Read the model definition and answer for the solid it produces. Units are mm, in the model's axes. A direction names the side the tool comes from. Coordinates: 2 decimals unless noted, no trailing zeros. Write each loop counter-clockwise with the first axis right and the second up, starting at its lowest first coordinate (ties: lowest second). Pieces come first, ordered by that corner, then holes.
1) Determine the mould class of faces 1 (the face through (0, 11, -17.5)), 2 (the face through (15.32, 3.62, 13.75)), 3 (the face through (-4.29, 13, 15)), 4 (the face through (-15, 13, 10.015)) for opening direction X: +X half, -X half, draft (parallel to the pull), parting line (faces both ways), or undercut.
2) The part is cut by section D-D (y = 13). Determine the outline of the cut face in (x, z), then the cut area to 3 significant figures.
3) The part is cut by section C-C (x = 4). Determine the outline of the cut face in (y, z).
4) Each of these flat-tipped pins is pushed along its axis until it touches: pin 1 Ø2.5 at (x, z) = (-15.25, 15.25) entering from +Y (3 decimals); pin 2 Ø1.8 at (x, y) = (-19, 0.5) entering from -Z; pin 3 Ø1 at (y, z) = (13, -15.5) entering from +X; pin 4 Ø0.6 at (x, y) = (-6.5, 1) entering from +Z. Where does it stop, or does it pass through?
5) Find the intervals of material crossed by line 1 (X direction, y = 8.75, z = 15.25); line 2 (Y direction, x = 18, z = 14); line 3 (Y direction, x = 5, z = -9), in increasing order.
6) Which of the six approach directions +Z, -Z, +X, -X, +Y, -Y give full straight-line access (tool end or side, diameter ignored) to faces 5 (the face through (-19, 1, -15.25)), 6 (the face through (1, 13, -0.479)), 7 (the face through (1, 13, -10.493)), 8 (the face through (-13.972, 13, 7)), 9 (the face through (-9, 13, 13.604))?
7) The part is cut by section B-B (z = -3). Determine the outline of the cut face in (x, y), then the cut area to 3 significant figures.
8) The part is cut by section A-A (y = 4). Determine the outline of the cut face in (x, z), then the cut area to 3 significant figures.
from build123d import *

# Parameters (mm, degrees)
EXTRUDE_1_DEPTH     = 2
SKETCH_2_R          = 2.5
EXTRUDE_2_DEPTH     = 5
EXTRUDE_START       = 8
SKETCH_3_R          = 2.5
EXTRUDE_3_DEPTH     = 8
EXTRUDE_4_DEPTH     = 2
CUT_EXTRUDE_1_DEPTH = 2
FILLET_1_R          = 2
SKETCH_6_W          = 8.710152629
SKETCH_6_H          = 2.597522262
SKETCH_6_W_2        = 2.966490945
SKETCH_6_H_2        = 5.729895294
SKETCH_6_W_3        = 8.81583313
SKETCH_6_H_3        = 2.597522261
SKETCH_6_W_4        = 9.797596015
SKETCH_6_H_4        = 10.014261194
EXTRUDE_5_DEPTH     = 2
SKETCH_7_R          = 1.5
CUT_EXTRUDE_2_DEPTH = 36.146123542


with BuildPart() as part:
    # 草图1 → 凸台-拉伸1 (new body)
    with BuildSketch(Plane(origin=(0, 0, 0), x_dir=(1, 0, 0), z_dir=(0, 1, 0))):
        Polygon((-21.5, -22), (-19.5, -22), (-19.5, -23), (19.5, -23), (19.5, -22), (21.5, -22), (21.5, 22), (-21.5, 22), align=None)
    extrude(amount=EXTRUDE_1_DEPTH)

    # 草图2 → 凸台-拉伸2 (add)
    with BuildSketch(Plane.XZ):
        with Locations(Location((-15.25, 15.25, 0), (0, 0, 90))):
            Circle(SKETCH_2_R)
        with Locations(Location((15.25, 15.25, 0), (0, 0, 90))):
            Circle(SKETCH_2_R)
        with Locations(Location((15.25, -15.25, 0), (0, 0, 90))):
            Circle(SKETCH_2_R)
        with Locations(Location((-15.25, -15.25, 0), (0, 0, 90))):
            Circle(SKETCH_2_R)
    extrude(amount=EXTRUDE_2_DEPTH)

    # 草图3 → 凸台-拉伸3 (add)
    with BuildSketch(Plane(origin=(0, 2, 0), x_dir=(1, 0, 0), z_dir=(0, 1, 0)).offset(EXTRUDE_START)):
        with Locations(Location((-15.25, 15.25, 0), (0, 0, 270))):
            Circle(SKETCH_3_R)
        with Locations(Location((15.25, 15.25, 0), (0, 0, 270))):
            Circle(SKETCH_3_R)
        with Locations(Location((15.25, -15.25, 0), (0, 0, 270))):
            Circle(SKETCH_3_R)
        with Locations(Location((-15.25, -15.25, 0), (0, 0, 270))):
            Circle(SKETCH_3_R)
    extrude(amount=-EXTRUDE_3_DEPTH)

    # 草图4 → 凸台-拉伸4 (add)
    with BuildSketch(Plane(origin=(0, 10, 0), x_dir=(1, 0, 0), z_dir=(0, 1, 0))):
        with BuildLine():
            Line((-13, 17.5), (13, 17.5))
            ThreePointArc((13, 17.5), (17.5, 17.5), (17.5, 13))
            Line((17.5, 13), (17.5, -13))
            ThreePointArc((17.5, -13), (17.5, -17.5), (13, -17.5))
            Line((13, -17.5), (-13, -17.5))
            ThreePointArc((-13, -17.5), (-17.5, -17.5), (-17.5, -13))
            Line((-17.5, -13), (-17.5, 13))
            ThreePointArc((-17.5, 13), (-17.5, 17.5), (-13, 17.5))
        make_face()
    extrude(amount=EXTRUDE_4_DEPTH)

    # 草图5 → 切除-拉伸1 (cut)
    with BuildSketch(Plane.XZ):
        with BuildLine():
            Line((15.25, 17.85), (-15.25, 17.85))
            ThreePointArc((-15.25, 17.85), (-17.088477631, 17.088477631), (-17.85, 15.25))
            Line((-17.85, 15.25), (-21.5, 15.25))
            Line((-21.5, 15.25), (-21.5, 22))
            Line((-21.5, 22), (-19.5, 22))
            Line((-19.5, 22), (-19.5, 23))
            Line((-19.5, 23), (19.5, 23))
            Line((19.5, 23), (19.5, 22))
            Line((19.5, 22), (21.5, 22))
            Line((21.5, 22), (21.5, 15.25))
            Line((21.5, 15.25), (17.85, 15.25))
            ThreePointArc((17.85, 15.25), (17.088477631, 17.088477631), (15.25, 17.85))
        make_face()
        with BuildLine():
            Line((21.5, -15.25), (17.85, -15.25))
            ThreePointArc((17.85, -15.25), (17.088477631, -17.088477631), (15.25, -17.85))
            Line((15.25, -17.85), (15.25, -22))
            Line((15.25, -22), (21.5, -22))
            Line((21.5, -22), (21.5, -15.25))
        make_face()
        with BuildLine():
            Line((-21.5, -15.25), (-17.85, -15.25))
            ThreePointArc((-17.85, -15.25), (-17.088477631, -17.088477631), (-15.25, -17.85))
            Line((-15.25, -17.85), (-15.25, -22))
            Line((-15.25, -22), (-21.5, -22))
            Line((-21.5, -22), (-21.5, -15.25))
        make_face()
    extrude(amount=-CUT_EXTRUDE_1_DEPTH, mode=Mode.SUBTRACT)

    # 圆角1
    fillet_1_edges = [part.edges().sort_by_distance(p)[0] for p in [
        (-21.5, 1, 15.25),
        (21.5, 1, 15.25),
        (21.5, 1, -15.25),
        (15.25, 1, -22),
        (-21.5, 1, -15.25),
        (-15.25, 1, -22),
    ]]
    fillet(fillet_1_edges, radius=FILLET_1_R)

    # 草图6 → 凸台-拉伸5 (add)
    with BuildSketch(Plane(origin=(0, 12, 0), x_dir=(1, 0, 0), z_dir=(0, 1, 0))):
        with Locations((-8.644923686, 15.086472233)):
            Rectangle(SKETCH_6_W, SKETCH_6_H)
        with Locations((-15.454766728, -7.149892581)):
            Rectangle(SKETCH_6_W_2, SKETCH_6_H_2)
        with Locations((-8.697763936, -14.903102968)):
            Rectangle(SKETCH_6_W_3, SKETCH_6_H_3)
        with Locations((1.034483131, 5.486228782)):
            Rectangle(SKETCH_6_W_4, SKETCH_6_H_4)
    extrude(amount=EXTRUDE_5_DEPTH)

    # 草图7 → 切除-拉伸2 (cut, through all)
    with BuildSketch(Plane(origin=(0, 12, 0), x_dir=(1, 0, 0), z_dir=(0, 1, 0))):
        with Locations(Location((-15.25, 15.25, 0), (0, 0, 270))):
            Circle(SKETCH_7_R)
        with Locations(Location((15.25, 15.25, 0), (0, 0, 270))):
            Circle(SKETCH_7_R)
        with Locations(Location((15.25, -15.25, 0), (0, 0, 270))):
            Circle(SKETCH_7_R)
        with Locations(Location((-15.25, -15.25, 0), (0, 0, 270))):
            Circle(SKETCH_7_R)
    extrude(amount=-CUT_EXTRUDE_2_DEPTH, mode=Mode.SUBTRACT)


solid = part.part
Reported:
1. face 1: undercut
1. face 2: undercut
1. face 3: +X half
1. face 4: draft
2. outline: (-16.94, 4.28) - (-13.97, 4.28) - (-13.97, 10.01) - (-16.94, 10.01) - close; (-13.11, 13.6) - (-4.29, 13.6) - (-4.29, 16.2) - (-13.11, 16.2) - close; (-13, -16.39) - (-4.29, -16.39) - (-4.29, -13.79) - (-13, -13.79) - close; (-3.86, -10.49) - (5.93, -10.49) - (5.93, -0.48) - (-3.86, -0.48) - close
2. area: 161 mm2
3. outline: (0, -22) - (2, -22) - (2, 17.85) - (0, 17.85) - close; (10, -17.5) - (12, -17.5) - (12, -10.49) - (14, -10.49) - (14, -0.48) - (12, -0.48) - (12, 17.5) - (10, 17.5) - close
4. pin 1: passes through
4. pin 2: stops at z = -15.25
4. pin 3: stops at x = -4.29
4. pin 4: stops at z = 17.85
5. line 1: x = -17.75 to -16.75, -13.75 to -12.75, 12.75 to 13.75, 16.75 to 17.75
5. line 2: y = 0 to 2, 10 to 12
5. line 3: y = 0 to 2, 10 to 14
6. face 5: -Z, -X, -Y
6. face 6: +Z, +X, -X, +Y
6. face 7: -Z, +X, -X, +Y
6. face 8: +Z, -Z, +X, +Y
6. face 9: +X, -X, +Y
7. outline: (-21.5, 0) - (21.5, 0) - (21.5, 2) - (-21.5, 2) - close; (-17.5, 10) - (17.5, 10) - (17.5, 12) - (5.93, 12) - (5.93, 14) - (-3.86, 14) - (-3.86, 12) - (-17.5, 12) - close
7. area: 176 mm2
8. outline: circle Ø5 at (-15.25, -15.25); circle Ø5 at (-15.25, 15.25); circle Ø5 at (15.25, -15.25); circle Ø5 at (15.25, 15.25); hole circle Ø3 at (-15.25, -15.25); hole circle Ø3 at (-15.25, 15.25); hole circle Ø3 at (15.25, -15.25); hole circle Ø3 at (15.25, 15.25)
8. area: 50.3 mm2
